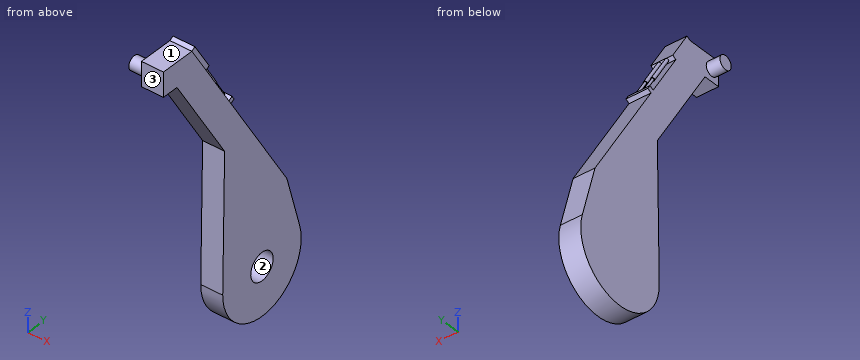
from build123d import *

# Parameters (mm, degrees)
BOSS_EXTRUDE1_DEPTH = 80
SKETCH2_R           = 50
CUT_EXTRUDE1_DEPTH  = 60
SKETCH3_R           = 25
BOSS_EXTRUDE2_DEPTH = 50
SKETCH4_W           = 79.742563162
SKETCH4_H           = 121.394874173
SKETCH4_W_2         = 80.091391525
SKETCH4_H_2         = 17.848004333
BOSS_EXTRUDE3_DEPTH = 16
SKETCH5_R           = 4.240124883
BOSS_EXTRUDE4_DEPTH = 73
SKETCH6_R           = 6
BOSS_EXTRUDE5_DEPTH = 130


with BuildPart() as part:
    # Sketch1 → Boss-Extrude1 (new body)
    with BuildSketch(Plane(origin=(0, 0, 0), x_dir=(0, 0, -1), z_dir=(1, 0, 0))):
        with BuildLine():
            Line((331.735644451, 300.452842372), (135.556846967, 243.860961507))
            Line((135.556846967, 243.860961507), (-555.240216811, -180.334724))
            Line((-555.240216811, -180.334724), (-555.240216811, -307.30913461))
            Line((-555.240216811, -307.30913461), (-466.406773101, -307.30913461))
            Line((-466.406773101, -307.30913461), (-466.406773101, -246.770086346))
            Line((-466.406773101, -246.770086346), (-120.382687357, -34.288111609))
            Line((-120.382687357, -34.288111609), (380.240216811, -42.69086539))
            ThreePointArc((380.240216811, -42.69086539), (553.517666092, 156.80251271), (331.735644451, 300.452842372))
        make_face()
    extrude(amount=BOSS_EXTRUDE1_DEPTH)

    # Sketch2 → Cut-Extrude1 (cut)
    with BuildSketch(Plane(origin=(80, 0, 0), x_dir=(0, 0, -1), z_dir=(1, 0, 0))):
        with Locations((380.240216811, 132.30913461)):
            Circle(SKETCH2_R)
    extrude(amount=-CUT_EXTRUDE1_DEPTH, mode=Mode.SUBTRACT)

    # Sketch3 → Boss-Extrude2 (add)
    with BuildSketch(Plane.ZY):
        with Locations(Location((510.240216811, -277.30913461, 0), (0, 0, 180))):
            Circle(SKETCH3_R)
    extrude(amount=BOSS_EXTRUDE2_DEPTH)

    # Sketch4 → Boss-Extrude3 (add)
    with BuildSketch(Plane(origin=(0, 116.638229969, 71.623688797), x_dir=(1, 0, 0), z_dir=(0, 0.8521590965506678, 0.5232827860401582))):
        with Locations((39.871281581, -506.821621235)):
            Rectangle(SKETCH4_W, SKETCH4_H)
        with Locations((40.045695763, -243.31556705)):
            Rectangle(SKETCH4_W_2, SKETCH4_H_2)
    extrude(amount=BOSS_EXTRUDE3_DEPTH)

    # Sketch5 → Boss-Extrude4 (add)
    with BuildSketch(Plane(origin=(0, -131.992624529, 214.948243417), x_dir=(1, 0, 0), z_dir=(0, -0.5232827860401582, 0.8521590965506678))):
        with Locations(Location((26.380961451, 146.454280366, 0), (0, 0, 90))):
            Circle(SKETCH5_R)
        with Locations(Location((53.361601711, 146.454280366, 0), (0, 0, 90))):
            Circle(SKETCH5_R)
    extrude(amount=BOSS_EXTRUDE4_DEPTH)

    # Sketch6 → Boss-Extrude5 (add)
    with BuildSketch(Plane(origin=(0, -170.19226791, 277.155857465), x_dir=(1, 0, 0), z_dir=(0, -0.5232827860401582, 0.8521590965506676))):
        with Locations(Location((26.380961451, 146.454280366, 0), (0, 0, 270))):
            Circle(SKETCH6_R)
        with Locations(Location((53.361601711, 146.454280366, 0), (0, 0, 270))):
            Circle(SKETCH6_R)
    extrude(amount=BOSS_EXTRUDE5_DEPTH)


solid = part.part
Read the model definition and answer for the solid it produces. Units are mm, in the model's axes. Face numbers are marked on the shaded views. Round coordinates to 2 decimals unless told otherwise and drop trailing zeros. Loops run counter-clockwise (first coordinate to the right, second up) from the corner with the lowest first, then second, coordinate; pieces in that order, holes last.
Q1. Each of these flat-tipped pins is pushed along its axis until it touches: pin 1 (12 mm diameter, centred on x = -4.5, y = -158.5, fed in from +Z); pin 2 (6 mm diameter, centred on y = -13, z = 5.5, fed in from +X); pin 3 (10 mm diameter, centred on x = 57, y = 58.5, fed in from +Z). Where does it stop, or does it pass through?
Q2. Section B-B on z = -488 is taken. Write down the section's boundary in (x, y), and give its area (3 significant figures).
Q3. Consider probe 1 along Y at (x, z) = (6, -384); probe 2 along Z at (x, y) = (55, -65.5); probe 3 along Y at (x, z) = (56, -398.5). Determine where each line is inside the solid, lowest interval first.
Q4. Section A-A on y = 46.5 is taken. Write down the section's boundary in (x, z), and give its area (3 significant figures).
Q5. Determine the mould class of the marked faces 1, 2 and 3 for opening direction Z: released by +Z, released by -Z, zero draft, split by the parting line, or undercut.
Q6. Section C-C on x = -15.5 is taken. Write down the section's boundary in (y, z), and give its area (3 significant figures).
Q7. Section D-D on y = -141.5 is taken. Write down the section's boundary in (x, z).
Output:
1. pin 1: stops at z = 556.72
1. pin 2: stops at x = 80
1. pin 3: stops at z = 174.44
2. outline: (0, -5.58) - (80, -5.58) - (80, 270.2) - (0, 270.2) - close
2. area: 22,100 mm2
3. probe 1: y = -42.65 to 307.27
3. probe 2: z = 171.21 to 368.23, 375.51 to 397.57
3. probe 3: y = -41.74 to 85.76, 178.86 to 306.35
4. outline: (0, -532.76) - (80, -532.76) - (80, 185.84) - (0, 185.84) - close
4. area: 57,500 mm2
5. face 1: released by +Z
5. face 2: undercut
5. face 3: zero draft
6. outline: circle Ø50 at (-277.31, 510.24)
6. area: 1,960 mm2
7. outline: (0, 294.98) - (80, 294.98) - (80, 492) - (79.74, 492) - (79.74, 522.57) - (0, 522.57) - close
